Verification items for the finished model (mm, model axes). A direction names the side the tool comes from. Give positions to 0.01 mm unless a question says otherwise; leave off trailing zeros. Write each loop counter-clockwise with the first axis right and the second up, starting at its lowest first coordinate (ties: lowest second). Pieces come first, ordered by that corner, then holes.
from build123d import *

# Parameters (mm, degrees)
SKETCH1_W                 = 30
SKETCH1_H                 = 40
BOSS_EXTRUDE1_DEPTH       = 1
SKETCH4_W                 = 1
SKETCH4_H                 = 44
BOSS_EXTRUDE2_DEPTH       = 9
SKETCH5_R                 = 1.1
CUT_EXTRUDE1_DEPTH        = 1
F_2_0MM_DOWEL_HOLE1_D     = 2
F_2_0MM_DOWEL_HOLE1_DEPTH = 2.6
F_2_0MM_DOWEL_HOLE1_TIP   = 0.600860619
FILLET3_R                 = 3


with BuildPart() as part:
    # Sketch1 → Boss-Extrude1 (new body)
    with BuildSketch(Plane(origin=(0, 0, 0), x_dir=(1, 0, 0), z_dir=(0, 1, 0))):
        with Locations((-15, 0)):
            Rectangle(SKETCH1_W, SKETCH1_H)
    extrude(amount=BOSS_EXTRUDE1_DEPTH)

    # Sketch4 → Boss-Extrude2 (add)
    with BuildSketch(Plane(origin=(0, 0, 0), x_dir=(1, 0, 0), z_dir=(0, 1, 0))):
        with Locations((-0.5, 0)):
            Rectangle(SKETCH4_W, SKETCH4_H)
    extrude(amount=BOSS_EXTRUDE2_DEPTH)

    # Sketch5 → Cut-Extrude1 (cut)
    with BuildSketch(Plane(origin=(0, 0, 0), x_dir=(0, 0, -1), z_dir=(1, 0, 0))):
        with Locations((-19, 6)):
            Circle(SKETCH5_R)
        with Locations((19, 6)):
            Circle(SKETCH5_R)
        with Locations((0, 5)):
            Circle(SKETCH5_R)
    extrude(amount=-CUT_EXTRUDE1_DEPTH, mode=Mode.SUBTRACT)

    # Ø2.0mm Dowel Hole1
    with Locations(Plane(origin=(0, 0, 0), x_dir=(-1, 0, 0), z_dir=(0, -1, 0))):
        with Locations((27.29, -16.3), (27.29, 16.3)):
            Hole(F_2_0MM_DOWEL_HOLE1_D / 2, depth=F_2_0MM_DOWEL_HOLE1_DEPTH)
            with Locations((0, 0, -(F_2_0MM_DOWEL_HOLE1_DEPTH + F_2_0MM_DOWEL_HOLE1_TIP / 2))):  # 118° drill point
                Cone(0, F_2_0MM_DOWEL_HOLE1_D / 2, F_2_0MM_DOWEL_HOLE1_TIP, mode=Mode.SUBTRACT)

    # Fillet3
    fillet3_edges = [part.edges().sort_by_distance(p)[0] for p in [
        (-0.5, 9, -22),
        (-0.5, 9, 22),
    ]]
    fillet(fillet3_edges, radius=FILLET3_R)


solid = part.part
Item 1: Scan lines: line 1 along Z through (x, y) = (-27.29, 0.75); line 2 along X through (y, z) = (0.55, 16.3); line 3 along Y through (x, z) = (-0.25, 0). Record each from-to range of solid material in increasing order.
Answer key:
line 1: z = -20 to -17.3, -15.3 to 15.3, 17.3 to 20
line 2: x = -30 to -28.29, -26.29 to 0
line 3: y = 0 to 3.9, 6.1 to 9
Item 2: Depth check by flat-ended pin: pin 1 (1.8 mm diameter, centred on y = 5, z = 0, fed in from +X) (1 decimal); pin 2 (1.1 mm diameter, centred on x = -13, y = 0.5, fed in from +Z); pin 3 (1.5 mm diameter, centred on x = -18, z = -14, fed in from +Y); pin 4 (3 mm diameter, centred on y = 4, z = 13, fed in from -X). Enter the tip coordinate at first touch or a pass-through.
Answer key:
pin 1: passes through
pin 2: stops at z = 20
pin 3: stops at y = 1
pin 4: stops at x = -1
Item 3: Sectioned sample at B-B on x = -27.29. Record the cut outline in (y, z).
Answer key:
outline: (0, -20) - (1, -20) - (1, -17.3) - (0, -17.3) - close; (0, -15.3) - (1, -15.3) - (1, 15.3) - (0, 15.3) - close; (0, 17.3) - (1, 17.3) - (1, 20) - (0, 20) - close
Item 4: Sectioned sample at C-C on z = 0. Record the cut outline in (x, y).
Answer key:
outline: (-30, 0) - (0, 0) - (0, 3.9) - (-1, 3.9) - (-1, 1) - (-30, 1) - close; (-1, 6.1) - (0, 6.1) - (0, 9) - (-1, 9) - close
Item 5: Sectioned sample at D-D on y = 2. Record the cut outline in (x, z).
Answer key:
outline: (-1, -22) - (0, -22) - (0, 22) - (-1, 22) - close
Item 6: Set-up check for faces 4 (the face through (-15.7, 0.5, -20)), 5 (the face through (-15.7, 0.5, 20)), 6 (the face through (-0.5, 6, -17.9)), 7 (the face through (-26.366, 0.507, 16.683)), 8 (the face through (-16, 1, 0)): record each of +Z, -Z, +X, -X, +Y, -Y from which the full face is reachable in a straight line by a thin tool's end or side.
Answer key:
face 4: -Z, -X, +Y, -Y
face 5: +Z, -X, +Y, -Y
face 6: +X, -X
face 7: +Y, -Y
face 8: +Z, -Z, -X, +Y
Item 7: Release check for a two-part mould opening along Y. For faces 1 (the face through (-0.5, 6, 20.1)), 2 (the face through (-0.5, 9, -0.3)), 3 (the face through (-15, 0, 0)) record: released by +Y, released by -Y, zero draft, split by the parting line, or undercut.
Answer key:
face 1: undercut
face 2: released by +Y
face 3: released by -Y
Item 8: Sectioned sample at A-A on z = -16.3. Record the cut outline in (x, y), then the cut area to 3 significant figures.
Answer key:
outline: (-30, 0) - (-28.29, 0) - (-28.29, 1) - (-30, 1) - close; (-26.29, 0) - (0, 0) - (0, 9) - (-1, 9) - (-1, 1) - (-26.29, 1) - close
area: 36.0 mm2
